Design review of the part built by this model. Coordinates are the model's own, in mm. Face numbers are marked on the shaded views. A direction names the side the tool comes from. Coordinates: 2 decimals unless noted, no trailing zeros. Write each loop counter-clockwise with the first axis right and the second up, starting at its lowest first coordinate (ties: lowest second). Pieces come first, ordered by that corner, then holes. Notation, with made-up numbers: (41.25, 27.25) - (81.25, 27.25) arc R6 cw to (81.25, 35.25) - close; hole circle Ø6 at (-1.75, 27.5). An arc over 180 degrees is marked (long way). One line per item, written item: value.
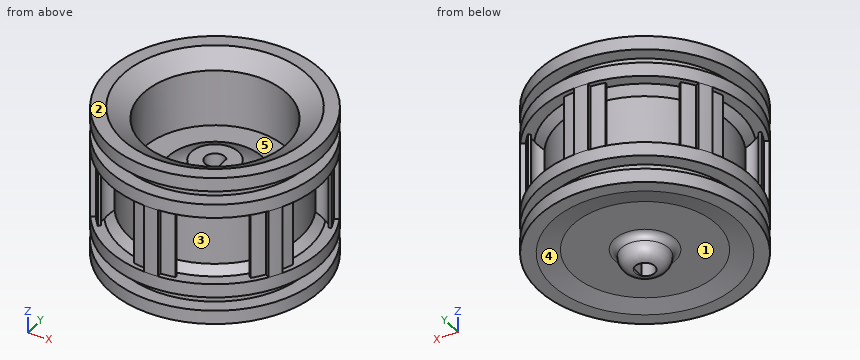
from build123d import *
from build123d.topology import SkipClean

# Parameters (mm, degrees)
EXTRUDE_1_DEPTH = 5
EXTRUDE_2_DEPTH = 16.5


with BuildPart() as part:
    # Эскиз2 → Повернуть1 (revolve)
    with BuildSketch(Plane(origin=(0, 0, 0), x_dir=(0, 0, -1), z_dir=(1, 0, 0)), mode=Mode.PRIVATE) as revolve_1_sk:
        with BuildLine():
            Line((4, 12.5), (-4, 12.5))
            Line((-4, 12.5), (-5, 13.799038106))
            Line((-5, 13.799038106), (-5, 15.5))
            Line((-5, 15.5), (-7, 15.5))
            Line((-7, 15.5), (-7, 13.5))
            Line((-7, 13.5), (-9, 13.5))
            Line((-9, 13.5), (-9, 15.5))
            Line((-9, 15.5), (-11, 15.5))
            Line((-11, 15.5), (-11, 13.5))
            Line((-11, 13.5), (-9.267949192, 10.5))
            Line((-9.267949192, 10.5), (-1.003318646, 10.5))
            Line((-1.003318646, 10.5), (-1.003318646, 6.908353552))
            Line((-1.003318646, 6.908353552), (-3, 3.45))
            Line((-3, 3.45), (-3, 1.45))
            Line((-3, 1.45), (10.5, 1.45))
            Line((10.5, 1.45), (13.5, 1.45))
            ThreePointArc((13.5, 1.45), (12.914213562, 2.864213562), (11.5, 3.45))
            ThreePointArc((11.5, 3.45), (10.792893219, 3.742893219), (10.5, 4.45))
            Line((10.5, 4.45), (10.5, 10.5))
            Line((10.5, 10.5), (11, 13.5))
            Line((11, 13.5), (11, 15.5))
            Line((11, 15.5), (9, 15.5))
            Line((9, 15.5), (9, 13.5))
            Line((9, 13.5), (7, 13.5))
            Line((7, 13.5), (7, 15.5))
            Line((7, 15.5), (5, 15.5))
            Line((5, 15.5), (5, 13.799038106))
            Line((5, 13.799038106), (4, 12.5))
        make_face()
    revolve(revolve_1_sk.sketch.rotate(Axis((0, 0, 12.144486905), (0, 0, -1)), 90), axis=Axis((0, 0, 12.144486905), (0, 0, -1)))

    # Эскиз4 → Бобышка-Вытянуть1 (add, symmetric)
    with SkipClean():  # the faces are left unmerged after this step: merging them gives an invalid solid
        with BuildSketch(Plane.XY):
            with BuildLine():
                Line((-1, 15.467708298), (-1, 14.766177569))
                ThreePointArc((-1, 14.766177569), (-2.004666987, 14.663604955), (-3, 14.492756812))
                Line((-3, 14.492756812), (-2.921430328, 14.113193095))
                ThreePointArc((-2.921430328, 14.113193095), (-1.553920806, 13.759344463), (-1, 12.459935794))
                ThreePointArc((-1, 12.459935794), (0, 12.5), (1, 12.459935794))
                ThreePointArc((1, 12.459935794), (1.553920806, 13.759344463), (2.921430328, 14.113193095))
                Line((2.921430328, 14.113193095), (3, 14.492756812))
                ThreePointArc((3, 14.492756812), (2.004666987, 14.663604955), (1, 14.766177569))
                Line((1, 14.766177569), (1, 15.467708298))
                ThreePointArc((1, 15.467708298), (0, 15.5), (-1, 15.467708298))
            make_face()
            with BuildLine():
                Line((12.895428325, 8.599879553), (12.287884892, 8.249114188))
                ThreePointArc((12.287884892, 8.249114188), (11.696720909, 9.067895014), (11.05109557, 9.844454617))
                Line((11.05109557, 9.844454617), (10.761668585, 9.586629427))
                ThreePointArc((10.761668585, 9.586629427), (11.138981441, 8.225407125), (10.290620927, 7.095993301))
                ThreePointArc((10.290620927, 7.095993301), (10.825317547, 6.25), (11.290620927, 5.363942493))
                ThreePointArc((11.290620927, 5.363942493), (12.692902247, 5.533937338), (13.683098913, 4.526563668))
                Line((13.683098913, 4.526563668), (14.05109557, 4.648302194))
                ThreePointArc((14.05109557, 4.648302194), (13.701387895, 5.595709941), (13.287884892, 6.517063381))
                Line((13.287884892, 6.517063381), (13.895428325, 6.867828745))
                ThreePointArc((13.895428325, 6.867828745), (13.423393759, 7.75), (12.895428325, 8.599879553))
            make_face()
            with BuildLine():
                Line((13.895428325, -6.867828745), (13.287884892, -6.517063381))
                ThreePointArc((13.287884892, -6.517063381), (13.701387895, -5.595709941), (14.05109557, -4.648302194))
                Line((14.05109557, -4.648302194), (13.683098913, -4.526563668))
                ThreePointArc((13.683098913, -4.526563668), (12.692902247, -5.533937338), (11.290620927, -5.363942493))
                ThreePointArc((11.290620927, -5.363942493), (10.825317547, -6.25), (10.290620927, -7.095993301))
                ThreePointArc((10.290620927, -7.095993301), (11.138981441, -8.225407125), (10.761668585, -9.586629427))
                Line((10.761668585, -9.586629427), (11.05109557, -9.844454617))
                ThreePointArc((11.05109557, -9.844454617), (11.696720909, -9.067895014), (12.287884892, -8.249114188))
                Line((12.287884892, -8.249114188), (12.895428325, -8.599879553))
                ThreePointArc((12.895428325, -8.599879553), (13.423393759, -7.75), (13.895428325, -6.867828745))
            make_face()
            with BuildLine():
                Line((1, -15.467708298), (1, -14.766177569))
                ThreePointArc((1, -14.766177569), (2.004666987, -14.663604955), (3, -14.492756812))
                Line((3, -14.492756812), (2.921430328, -14.113193095))
                ThreePointArc((2.921430328, -14.113193095), (1.553920806, -13.759344463), (1, -12.459935794))
                ThreePointArc((1, -12.459935794), (0, -12.5), (-1, -12.459935794))
                ThreePointArc((-1, -12.459935794), (-1.553920806, -13.759344463), (-2.921430328, -14.113193095))
                Line((-2.921430328, -14.113193095), (-3, -14.492756812))
                ThreePointArc((-3, -14.492756812), (-2.004666987, -14.663604955), (-1, -14.766177569))
                Line((-1, -14.766177569), (-1, -15.467708298))
                ThreePointArc((-1, -15.467708298), (0, -15.5), (1, -15.467708298))
            make_face()
            with BuildLine():
                Line((-12.895428325, -8.599879553), (-12.287884892, -8.249114188))
                ThreePointArc((-12.287884892, -8.249114188), (-11.696720909, -9.067895014), (-11.05109557, -9.844454617))
                Line((-11.05109557, -9.844454617), (-10.761668585, -9.586629427))
                ThreePointArc((-10.761668585, -9.586629427), (-11.138981441, -8.225407125), (-10.290620927, -7.095993301))
                ThreePointArc((-10.290620927, -7.095993301), (-10.825317547, -6.25), (-11.290620927, -5.363942493))
                ThreePointArc((-11.290620927, -5.363942493), (-12.692902247, -5.533937338), (-13.683098913, -4.526563668))
                Line((-13.683098913, -4.526563668), (-14.05109557, -4.648302194))
                ThreePointArc((-14.05109557, -4.648302194), (-13.701387895, -5.595709941), (-13.287884892, -6.517063381))
                Line((-13.287884892, -6.517063381), (-13.895428325, -6.867828745))
                ThreePointArc((-13.895428325, -6.867828745), (-13.423393759, -7.75), (-12.895428325, -8.599879553))
            make_face()
            with BuildLine():
                Line((-13.895428325, 6.867828745), (-13.287884892, 6.517063381))
                ThreePointArc((-13.287884892, 6.517063381), (-13.701387895, 5.595709941), (-14.05109557, 4.648302194))
                Line((-14.05109557, 4.648302194), (-13.683098913, 4.526563668))
                ThreePointArc((-13.683098913, 4.526563668), (-12.692902247, 5.533937338), (-11.290620927, 5.363942493))
                ThreePointArc((-11.290620927, 5.363942493), (-10.825317547, 6.25), (-10.290620927, 7.095993301))
                ThreePointArc((-10.290620927, 7.095993301), (-11.138981441, 8.225407125), (-10.761668585, 9.586629427))
                Line((-10.761668585, 9.586629427), (-11.05109557, 9.844454617))
                ThreePointArc((-11.05109557, 9.844454617), (-11.696720909, 9.067895014), (-12.287884892, 8.249114188))
                Line((-12.287884892, 8.249114188), (-12.895428325, 8.599879553))
                ThreePointArc((-12.895428325, 8.599879553), (-13.423393759, 7.75), (-13.895428325, 6.867828745))
            make_face()
        extrude(amount=EXTRUDE_1_DEPTH, both=True)

    # Эскиз5 → Бобышка-Вытянуть2 (add, through all)
    with SkipClean():  # the faces are left unmerged after this step: merging them gives an invalid solid
        with BuildSketch(Plane.XY.offset(3)):
            with BuildLine():
                Line((1.1, 0.944722181), (1.1, -0.944722181))
                ThreePointArc((1.1, -0.944722181), (1.45, 0), (1.1, 0.944722181))
            make_face()
        extrude(amount=-EXTRUDE_2_DEPTH)


solid = part.part
1. For the marked faces 3, 4 and 5, list the 3-axis set-ups (+Z, -Z, +X, -X, +Y, -Y) from which the entire face can be reached by the end or side of a thin tool; tool diameter is ignored.
Answer block:
face 3: none
face 4: -Z
face 5: +Z
2. Mouldability with a two-part tool opening along Y and no side actions: class the marked faces 1 and 2 as released by +Y, released by -Y, zero draft, split by the parting line, or undercut.
Answer block:
face 1: undercut
face 2: zero draft
3. Wall thickness on line 1 along Y through (x, z) = (0, -4); line 2 along Z through (x, y) = (-7, -13); line 3 along Z through (x, y) = (-7, -2.5): over which ranges is each line inside the solid? List them lowest first.
Answer block:
line 1: y = -15.5 to -1.45, 1.45 to 15.5
line 2: z = -11 to -9, -7 to -5, 5 to 7, 9 to 11
line 3: z = -10.5 to 1
4. Insertion check: pin 1 Ø2 at (x, y) = (4, -2.5) entering from +Z; pin 2 Ø9.5 at (x, y) = (0, 3.5) entering from +Z; pin 3 Ø10 at (x, z) = (-7.5, -8.5) entering from +Y; pin 4 Ø17 at (x, y) = (-5, -2) entering from +Z. Each pin has a flat end and moves straight along its axis. Give the tip position at first contact, or say it passes through.
Answer block:
pin 1: stops at z = 2.85
pin 2: stops at z = 3
pin 3: stops at y = 15.29
pin 4: stops at z = 11
5. Consider section A-A, the plane z = -7.75. Write out the cut boundary in (x, y), then the cut area to 3 significant figures.
Answer block:
outline: circle Ø27 at (0, 0); hole (1.1, -0.94) - (1.1, 0.94) arc R1.45 ccw (long way) to start
area: 566 mm^2
